Design review of the part built by this model. Coordinates are the model's own, in mm. A direction names the side the tool comes from. Give positions to 0.01 mm unless a question says otherwise; leave off trailing zeros. Write each loop counter-clockwise with the first axis right and the second up, starting at its lowest first coordinate (ties: lowest second). Pieces come first, ordered by that corner, then holes. Notation, with made-up numbers: (74.25, 4.5) -> (112.25, 4.5) arc R16 ccw to (112.25, 23.5) -> close; hole circle Ø1 at (30.5, -10.5). An arc over 180 degrees is marked (long way). Use CSV: the item, a comma, the result in double quotes.
```python
from build123d import *

# Parameters (mm, degrees)
SKETCH_1_W              = 100
SKETCH_1_H              = 230
EXTRUDE_1_DEPTH         = 10
EXTRUDE_2_DEPTH         = 135
EXTRUDE_2_DEPTH_BACK    = 50
SKETCH_1_3_W            = 12
SKETCH_1_3_H            = 230
SKETCH_2_W              = 125
SKETCH_2_H              = 15
EXTRUDE_3_DEPTH         = 120
CUT_EXTRUDE_1_DEPTH     = 245.642596455
CHAMFER_2_SIZE          = 20
HOLE_WIZARD_3_D         = 21
HOLE_WIZARD_3_DEPTH     = 100
HOLE_WIZARD_M10_1_D     = 8.5
HOLE_WIZARD_M10_1_DEPTH = 24.5
HOLE_WIZARD_M10_1_TIP   = 2.553657631
HOLE_WIZARD_2_D         = 10.5
HOLE_WIZARD_2_DEPTH     = 100


with BuildPart() as part:
    # 草图1 → 凸台-拉伸1 (new body)
    with BuildSketch(Plane.XY):
        with Locations((50, 0)):
            Rectangle(SKETCH_1_W, SKETCH_1_H)
    extrude(amount=EXTRUDE_1_DEPTH)

    # 草图1<3> → 凸台-拉伸2 (add, two sides: drawn at the far end of the back side and taken through both)
    with BuildSketch(Plane.XY.offset(-EXTRUDE_2_DEPTH_BACK)):
        with Locations((-6, 0)):
            Rectangle(SKETCH_1_3_W, SKETCH_1_3_H)
    extrude(amount=EXTRUDE_2_DEPTH + EXTRUDE_2_DEPTH_BACK)

    # 草图2 → 凸台-拉伸3 (add)
    with BuildSketch(Plane(origin=(0, 0, 0), x_dir=(0, 0, -1), z_dir=(1, 0, 0))):
        with Locations((-72.5, -42.5)):
            Rectangle(SKETCH_2_W, SKETCH_2_H)
        with Locations((-72.5, 42.5)):
            Rectangle(SKETCH_2_W, SKETCH_2_H)
    extrude(amount=EXTRUDE_3_DEPTH)

    # 草图3 → 切除-拉伸1 (cut, through all)
    with BuildSketch(Plane(origin=(0, 50, 0), x_dir=(1, 0, 0), z_dir=(0, 1, 0))):
        with BuildLine():
            Line((120, -115.25), (75, -115.25))
            ThreePointArc((75, -115.25), (59.75, -100), (75, -84.75))
            Line((75, -84.75), (120, -84.75))
            ThreePointArc((120, -84.75), (135.25, -100), (120, -115.25))
        make_face()
    extrude(amount=-CUT_EXTRUDE_1_DEPTH, mode=Mode.SUBTRACT)

    # 倒角2
    chamfer_2_edges = [part.edges().sort_by_distance(p)[0] for p in [
        (120, 42.5, 10),
        (120, -42.5, 10),
    ]]
    chamfer(chamfer_2_edges, length=CHAMFER_2_SIZE - 0.0001)  # a hair under: the kernel refuses the full size

    # 孔3
    with Locations(Plane(origin=(0, 0, 0), x_dir=(0, 0, -1), z_dir=(1, 0, 0))):
        with Locations((-100, -90), (-100, 90)):
            Hole(HOLE_WIZARD_3_D / 2, depth=HOLE_WIZARD_3_DEPTH)

    # M10 螺纹孔1
    with Locations(Plane.XY.offset(10)):
        with Locations((25, -90), (75, -90), (75, 90), (25, 90), (75, 0), (25, 0)):
            Hole(HOLE_WIZARD_M10_1_D / 2, depth=HOLE_WIZARD_M10_1_DEPTH)
            with Locations((0, 0, -(HOLE_WIZARD_M10_1_DEPTH + HOLE_WIZARD_M10_1_TIP / 2))):  # 118° drill point
                Cone(0, HOLE_WIZARD_M10_1_D / 2, HOLE_WIZARD_M10_1_TIP, mode=Mode.SUBTRACT)

    # 孔2
    with Locations(Plane.ZY.offset(12)):
        with Locations((-25, 90), (-25, -90), (-25, 0)):
            Hole(HOLE_WIZARD_2_D / 2, depth=HOLE_WIZARD_2_DEPTH)


solid = part.part
```
(1) Take a section at A-A (x = 91). Write out the cut boundary in (y, z).
Established:
outline,"(-115, 0) -> (115, 0) -> (115, 10) -> (50, 10) -> (50, 84.75) -> (35, 84.75) -> (35, 10) -> (-35, 10) -> (-35, 84.75) -> (-50, 84.75) -> (-50, 10) -> (-115, 10) -> close; (-50, 115.25) -> (-35, 115.25) -> (-35, 135) -> (-50, 135) -> close; (35, 115.25) -> (50, 115.25) -> (50, 135) -> (35, 135) -> close"
(2) For line 1 along Y through (x, z) = (25, 3); line 2 along Y through (x, z) = (-7, -25); line 3 along Y through (x, z) = (64, 111), list the stretches that pass through material, from the lowest coordinate up. Write a range as [from, to].
Established:
line 1,"y = [-115, -94.25], [-85.75, -4.25], [4.25, 85.75], [94.25, 115]"
line 2,"y = [-115, -95.25], [-84.75, -5.25], [5.25, 84.75], [95.25, 115]"
line 3,"y = [-50, -35], [35, 50]"
(3) Take a section at C-C (z = -25). Write out the cut boundary in (x, y).
Established:
outline,"(-12, -115) -> (0, -115) -> (0, -95.25) -> (-12, -95.25) -> close; (-12, -84.75) -> (0, -84.75) -> (0, -5.25) -> (-12, -5.25) -> close; (-12, 5.25) -> (0, 5.25) -> (0, 84.75) -> (-12, 84.75) -> close; (-12, 95.25) -> (0, 95.25) -> (0, 115) -> (-12, 115) -> close"
(4) Clearance check with flat-ended pins moving along their axes: pin 1 (4 mm diameter, centred on x = 39, z = 56.5, fed in from -Y); pin 2 (3 mm diameter, centred on y = 10.5, z = -6.5, fed in from +X); pin 3 (4.5 mm diameter, centred on x = 90.5, y = 46, fed in from -Z). State where each tip first meets the part, or that it passes through.
Established:
pin 1,"stops at y = -50"
pin 2,"stops at x = 0"
pin 3,"stops at z = 0"
(5) Take a section at B-B (y = 0). Write out the cut boundary in (x, z).
Established:
outline,"(-12, -50) -> (0, -50) -> (0, -30.25) -> (-12, -30.25) -> close; (-12, -19.75) -> (0, -19.75) -> (0, 0) -> (20.75, 0) -> (20.75, 10) -> (0, 10) -> (0, 135) -> (-12, 135) -> close; (29.25, 0) -> (70.75, 0) -> (70.75, 10) -> (29.25, 10) -> close; (79.25, 0) -> (100, 0) -> (100, 10) -> (79.25, 10) -> close"
(6) Take a section at D-D (y = 90). Write out the cut boundary in (x, z), then the cut area to 3 significant figures.
Established:
outline,"(-12, -50) -> (0, -50) -> (0, -30.25) -> (-12, -30.25) -> close; (-12, -19.75) -> (0, -19.75) -> (0, 0) -> (20.75, 0) -> (20.75, 10) -> (0, 10) -> (0, 89.5) -> (-12, 89.5) -> close; (-12, 110.5) -> (0, 110.5) -> (0, 135) -> (-12, 135) -> close; (29.25, 0) -> (70.75, 0) -> (70.75, 10) -> (29.25, 10) -> close; (79.25, 0) -> (100, 0) -> (100, 10) -> (79.25, 10) -> close"
area,"2,670 mm2"
(7) Tool access review of faces 1 (the face through (28.132, 2.872, 4.93)), 2 (the face through (0, 82, 72)), 3 (the face through (97, -42, 84.75)): name each direction out of +Z, -Z, +X, -X, +Y, -Y from which nothing blocks a thin tool from reaching the whole face with its end or side.
Established:
face 1,"+Z, -Z"
face 2,"+Z, +X, +Y"
face 3,"+X, +Y, -Y"
(8) Mouldability with a two-part tool opening along Z and no side actions: class faces 4 (the face through (49, -82, 10)), 5 (the face through (59, 35, 73)), 6 (the face through (59.754, 42.605, 100.335)), 7 (the face through (98, -42, 115.25)) as +Z half, -Z half, draft (parallel to the pull), parting line (faces both ways), or undercut.
Established:
face 4,"+Z half"
face 5,"draft"
face 6,"undercut"
face 7,"undercut"
